Build history of the part. All positions in model axes, mm. Face numbers are marked on the shaded views. A direction names the side the tool comes from. Round coordinates to 2 decimals unless told otherwise and drop trailing zeros. Order: outer loops, then holes, each group sorted by start corner. A loop starts at its lowest first (then second) coordinate and runs counter-clockwise, first axis right, second up. Notation, with made-up numbers: M 4,15 L 29,15 A24 cw 29,53 Z; hole C 4,-13 d4. An arc over 180 degrees is marked long. Use CSV: the item, a comma, the result in double quotes.
from build123d import *

# Parameters (mm, degrees)
SKETCH1_W           = 203.2
SKETCH1_H           = 203.2
BOSS_EXTRUDE1_DEPTH = 2.54
SKETCH3_R           = 9.525
BOSS_EXTRUDE2_DEPTH = 12.7
SKETCH5_R           = 34.925
CUT_EXTRUDE2_DEPTH  = 145.244271983
SKETCH7_R           = 9.525
BOSS_EXTRUDE4_DEPTH = 53.0225
FILLET1_R           = 2.54
SKETCH8_R           = 40.005
SKETCH8_R_2         = 34.925
BOSS_EXTRUDE5_DEPTH = 25.4
FILLET2_R           = 2.54


with BuildPart() as part:
    # Sketch1 → Boss-Extrude1 (new body)
    with BuildSketch(Plane(origin=(0, 0, 0), x_dir=(1, 0, 0), z_dir=(0, 1, 0))):
        Rectangle(SKETCH1_W, SKETCH1_H)
    extrude(amount=BOSS_EXTRUDE1_DEPTH)

    # Sketch3 → Boss-Extrude2 (add)
    with BuildSketch(Plane(origin=(0, 2.54, 0), x_dir=(1, 0, 0), z_dir=(0, 1, 0))):
        with Locations(Location((57.15, 0, 0), (0, 0, 270))):
            Circle(SKETCH3_R)
    extrude(amount=BOSS_EXTRUDE2_DEPTH)

    # Sketch5 → Cut-Extrude2 (cut, through all)
    with BuildSketch(Plane(origin=(0, 2.54, 0), x_dir=(1, 0, 0), z_dir=(0, 1, 0))):
        with Locations(Location((-14.741985059, 0, 0), (0, 0, 270))):
            Circle(SKETCH5_R)
    extrude(amount=-CUT_EXTRUDE2_DEPTH, mode=Mode.SUBTRACT)

    # Sketch7 → Boss-Extrude4 (add)
    with BuildSketch(Plane(origin=(0, 2.54, 0), x_dir=(1, 0, 0), z_dir=(0, 1, 0))):
        with Locations(Location((-88.9, 76.2, 0), (0, 0, 90))):
            Circle(SKETCH7_R)
    boss_extrude4 = extrude(amount=BOSS_EXTRUDE4_DEPTH)

    # Mirror1: Boss-Extrude4 across plane
    add(boss_extrude4.mirror(Plane.XY))

    # Fillet1
    fillet1_edges = [part.edges().sort_by_distance(p)[0] for p in [
        (101.6, 1.27, 101.6),
    ]]
    fillet(fillet1_edges, radius=FILLET1_R)

    # Sketch8 → Boss-Extrude5 (add)
    with BuildSketch(Plane.XZ):
        with Locations(Location((-14.741985059, 0, 0), (0, 0, 90))):
            Circle(SKETCH8_R)
        with Locations(Location((-14.741985059, 0, 0), (0, 0, 90))):
            Circle(SKETCH8_R_2, mode=Mode.SUBTRACT)
    extrude(amount=BOSS_EXTRUDE5_DEPTH)

    # Fillet2
    fillet2_edges = [part.edges().sort_by_distance(p)[0] for p in [
        (57.15, 2.54, -9.525),
        (-88.9, 2.54, -66.675),
        (-88.9, 2.54, 66.675),
    ]]
    fillet(fillet2_edges, radius=FILLET2_R)


solid = part.part
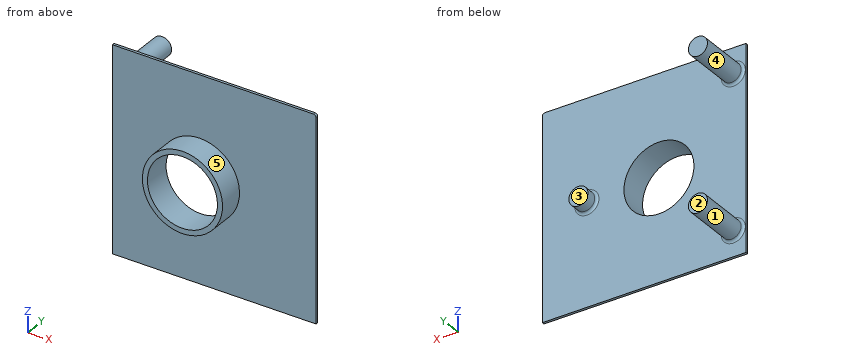
(1) Drop flat-ended pins along their axis: pin 1 (10 mm diameter, centred on y = 19, z = -70, fed in from -X); pin 2 (5.5 mm diameter, centred on x = 55, z = 3, fed in from +Y); pin 3 (10 mm diameter, centred on x = 32, z = 19, fed in from -Y). Give the stop position or say it passes through.
Answer block:
pin 1,"stops at x = -98.35"
pin 2,"stops at y = 15.24"
pin 3,"stops at y = 0"
(2) Tool access for the marked faces 1 and 2: list every direction of +Z, -Z, +X, -X, +Y, -Y with a clear straight run to the whole face (end or side of a thin tool).
Answer block:
face 1,"+Y"
face 2,"+Z, -Z, +X, -X, +Y"
(3) Wall check: line 1 (X direction, y = -14, z = 0); line 2 (Y direction, x = 38, z = -18); line 3 (Z direction, x = -34.5, y = -19). Give the ranges that are in metal, low to high. Write a range as from..to.
Answer block:
line 1,"x = -54.75..-49.67, 20.18..25.26"
line 2,"y = 0..2.54"
line 3,"z = -34.79..-28.8, 28.8..34.79"
(4) Cut at B-B, the plane x = 57.15. Give the cut face in (y, z) (3 decimals).
Answer block:
outline,"M 0,-101.6 L 2.54,-101.6 L 2.54,-12.065 A2.54 cw 5.08,-9.525 L 15.24,-9.525 L 15.24,9.525 L 5.08,9.525 A2.54 cw 2.54,12.065 L 2.54,101.6 L 0,101.6 Z"
(5) Two-plate mould, pull along Z, no slides. Class the marked faces 3, 4 and 5: released by +Z, released by -Z, zero draft, split by the parting line, or undercut.
Answer block:
face 3,"zero draft"
face 4,"undercut"
face 5,"split by the parting line"
(6) Cut at D-D, the plane x = -88.9. Give the cut face in (y, z) (1 decimal), and give its area (3 significant figures).
Answer block:
outline,"M 0,-101.6 L 2.5,-101.6 L 2.5,-88.3 A2.5 cw 5.1,-85.7 L 55.6,-85.7 L 55.6,-66.7 L 5.1,-66.7 A2.5 cw 2.5,-64.1 L 2.5,64.1 A2.5 cw 5.1,66.7 L 55.6,66.7 L 55.6,85.7 L 5.1,85.7 A2.5 cw 2.5,88.3 L 2.5,101.6 L 0,101.6 Z"
area,"2,540 mm²"
(7) Cut at A-A, the plane z = 0. Give the cut face in (x, y) (3 decimals).
Answer block:
outline,"M -101.6,0 L -54.747,0 L -54.747,-25.4 L -49.667,-25.4 L -49.667,2.54 L -101.6,2.54 Z; M 20.183,-25.4 L 25.263,-25.4 L 25.263,0 L 101.6,0 L 101.6,2.54 L 69.215,2.54 A2.54 cw 66.675,5.08 L 66.675,15.24 L 47.625,15.24 L 47.625,5.08 A2.54 cw 45.085,2.54 L 20.183,2.54 Z"
(8) Cut at C-C, the plane z = -76.2. Give the cut face in (x, y) (1 decimal), and give its area (3 significant figures).
Answer block:
outline,"M -101.6,0 L 101.6,0 L 101.6,2.5 L -76.8,2.5 A2.5 cw -79.4,5.1 L -79.4,55.6 L -98.4,55.6 L -98.4,5.1 A2.5 cw -101,2.5 L -101.6,2.5 Z"
area,"1,530 mm²"
